Input: part model. Units: mm. Frame: model coordinates. A direction names the side the tool comes from. Give positions to 0.01 mm unless a question says otherwise; leave off trailing zeros. Loops run counter-clockwise (first coordinate to the right, second up) from the corner with the lowest first, then second, coordinate; pieces in that order, holes last.
from build123d import *

# Parameters (mm, degrees)
F0_R      = 24.75
F1_DEPTH  = 20
F2_R      = 25
F3_DEPTH  = 16
F4_R      = 25
F5_DEPTH  = 16
F6_R      = 28
F7_DEPTH  = 21
F8_R      = 20
F9_DEPTH  = 55
F10_R     = 23.5
F11_DEPTH = 2
F12_R     = 25
F13_DEPTH = 20
F14_R     = 20
F15_DEPTH = 55


with BuildPart() as f1:
    # F0 (on Front) → F1 (new body)
    with BuildSketch(Plane.XZ):
        Circle(F0_R)
    extrude(amount=F1_DEPTH)

    # F2 (on face) → F3 (join)
    with BuildSketch(Plane.XZ.offset(20)):
        Circle(F2_R)
    extrude(amount=F3_DEPTH)

    # F4 (on face) → F5 (join)
    with BuildSketch(Plane(origin=(0, 0, 0), x_dir=(-1, 0, 0), z_dir=(0, 1, 0))):
        Circle(F4_R)
    extrude(amount=F5_DEPTH)

    # F6 (on face) → F7 (join)
    with BuildSketch(Plane.XZ.offset(36)):
        Circle(F6_R)
    extrude(amount=F7_DEPTH)

    # F8 (on face) → F9 (join)
    with BuildSketch(Plane.XZ.offset(57)):
        Circle(F8_R)
    extrude(amount=F9_DEPTH)

    # F10 (on face) → F11 (join)
    with BuildSketch(Plane(origin=(0, 16, 0), x_dir=(-1, 0, 0), z_dir=(0, 1, 0))):
        Circle(F10_R)
    extrude(amount=F11_DEPTH)

    # F12 (on face) → F13 (join)
    with BuildSketch(Plane(origin=(0, 18, 0), x_dir=(-1, 0, 0), z_dir=(0, 1, 0))):
        Circle(F12_R)
    extrude(amount=F13_DEPTH)

    # F14 (on face) → F15 (join)
    with BuildSketch(Plane(origin=(0, 38, 0), x_dir=(-1, 0, 0), z_dir=(0, 1, 0))):
        Circle(F14_R)
    extrude(amount=F15_DEPTH)


solid = f1.part
(1) Cut plane C-C (y = -92). Return the cut outline in (x, z).
Values follow:
outline: circle Ø40 at (0, 0)
(2) Pin query (flat end, axial travel): pin 1 Ø1.5 at (x, z) = (17, -15) entering from -Y; pin 2 Ø1.5 at (x, y) = (5, 51) entering from +Z; pin 3 Ø5 at (x, y) = (-9, 61.5) entering from -Z. Return the tip coordinate at first contact, or that it passes through.
Values follow:
pin 1: stops at y = -57
pin 2: stops at z = 19.54
pin 3: stops at z = -18.91
(3) Ray query, probe 1 along Y at (x, z) = (-17, 16.5); probe 2 along X at (y, z) = (47.5, 1); probe 3 along Y at (x, z) = (-23, 1.5). Return the intervals inside material, ascending.
Values follow:
probe 1: y = -57 to 16, 18 to 38
probe 2: x = -19.97 to 19.97
probe 3: y = -57 to 38
(4) Cut plane D-D (y = -5.5). Return the cut outline in (x, z), and give its area (3 significant figures).
Values follow:
outline: circle Ø49.5 at (0, 0)
area: 1,920 mm2
(5) Reachability of faces 1 (the cylindrical face through (-22.4, 17, 7.1)), 2 (the cylindrical face through (25.865, -46.353, -10.724)), 3 (the flat face through (0, -112, 0)), 4 (the cylindrical face through (-23.846, 27.86, 7.509)), 5 (the cylindrical face through (-4.336, -84.115, -19.524)) from +Z, -Z, +X, -X, +Y, -Y: full face, straight path, thin tool, end or side. Return the list, or none.
Values follow:
face 1: none
face 2: +Y, -Y
face 3: +Z, -Z, +X, -X, -Y
face 4: +Y
face 5: -Y
(6) Mould query, pull axis Y, two halves, no side actions, for faces 6 (the flat face through (17, 18, -17)), 7 (the flat face through (0, 93, 0)), 8 (the flat face through (-7, -57, 19)). Classes: +Y half, -Y half, draft (parallel to the pull), parting line (faces both ways), or undercut.
Values follow:
face 6: undercut
face 7: +Y half
face 8: -Y half
